```python
from build123d import *

# Parameters (mm, degrees)
EXTRUDE_1_DEPTH             = 8
EXTRUDE_9_DEPTH             = 29
SKETCH_25_W                 = 47
SKETCH_25_H                 = 36.5
EXTRUDE_10_DEPTH            = 4
HOLE_WIZARD_M51_D           = 3.2
HOLE_WIZARD_M51_CBORE_D     = 6
HOLE_WIZARD_M51_CBORE_DEPTH = 35
SKETCH_22_R                 = 2.6
CUT_EXTRUDE_9_DEPTH         = 92.536877814
CUT_EXTRUDE_10_DEPTH        = 4.2
HOLE_WIZARD_M52_D           = 5.2
HOLE_WIZARD_M52_CBORE_D     = 10
HOLE_WIZARD_M52_CBORE_DEPTH = 33
CUT_EXTRUDE_11_DEPTH        = 24
FILLET_1_R                  = 2.5
EXTRUDE_11_DEPTH            = 7
SKETCH_32_W                 = 15
SKETCH_32_H                 = 5.4
CUT_EXTRUDE_12_DEPTH        = 13.5
SKETCH_33_W                 = 15
SKETCH_33_H                 = 5.4
CUT_EXTRUDE_13_DEPTH        = 33.5


with BuildPart() as part:
    # Эскиз1 → Бобышка-Вытянуть1 (new body)
    with BuildSketch(Plane.XY):
        Polygon((-47, 51), (-47, 0), (0, 0), (0, 51), (-22, 51), (-22, 67), (-42, 67), (-42, 51), align=None)
    extrude(amount=EXTRUDE_1_DEPTH)

    # Эскиз24 → Бобышка-Вытянуть9 (add)
    with BuildSketch(Plane.XY.offset(8)):
        with BuildLine():
            Line((0, 51), (-3.5, 51))
            Line((-3.5, 51), (-3.5, 33.5))
            ThreePointArc((-3.5, 33.5), (-13.5, 23.5), (-23.5, 33.5))
            Line((-23.5, 33.5), (-23.5, 51))
            Line((-23.5, 51), (-47, 51))
            Line((-47, 51), (-47, 14.5))
            Line((-47, 14.5), (0, 14.5))
            Line((0, 14.5), (0, 51))
        make_face()
    extrude(amount=EXTRUDE_9_DEPTH)

    # Эскиз25 → Бобышка-Вытянуть10 (add)
    with BuildSketch(Plane.XY.offset(37)):
        with Locations((-23.5, 32.75)):
            Rectangle(SKETCH_25_W, SKETCH_25_H)
    extrude(amount=EXTRUDE_10_DEPTH)

    # Цековка для  болта с шестигранной головкой M51 (through all)
    with Locations(Plane(origin=(-33.5, 3.5, 41), x_dir=(1, 0, 0), z_dir=(0, 0, 1))):
        with Locations((0, 0), (0, 20), (20, 0), (20, 20)):
            CounterBoreHole(HOLE_WIZARD_M51_D / 2, HOLE_WIZARD_M51_CBORE_D / 2, HOLE_WIZARD_M51_CBORE_DEPTH)

    # Эскиз22 → Вырез-Вытянуть9 (cut, through all)
    with BuildSketch(Plane.XY):
        with Locations(Location((-13.5, 33.5, 0), (0, 0, 180))):
            Circle(SKETCH_22_R)
    extrude(amount=CUT_EXTRUDE_9_DEPTH, mode=Mode.SUBTRACT)

    # Эскиз23 → Вырез-Вытянуть10 (cut)
    with BuildSketch(Plane(origin=(0, 0, 0), x_dir=(-1, 0, 0), z_dir=(0, 0, -1))):
        Polygon((13.5, 38.234272207), (9.4, 35.867136104), (9.4, 31.132863896), (13.5, 28.765727793), (17.6, 31.132863896), (17.6, 35.867136104), align=None)
    extrude(amount=-CUT_EXTRUDE_10_DEPTH, mode=Mode.SUBTRACT)

    # Цековка для  болта с шестигранной головкой M52 (through all)
    with Locations(Plane(origin=(-32, 61.5, 41), x_dir=(1, 0, 0), z_dir=(0, 0, 1))):
        with Locations((0, 0), (0, -24.5)):
            CounterBoreHole(HOLE_WIZARD_M52_D / 2, HOLE_WIZARD_M52_CBORE_D / 2, HOLE_WIZARD_M52_CBORE_DEPTH)

    # Эскиз30 → Вырез-Вытянуть11 (cut)
    with BuildSketch(Plane(origin=(0, 51, 0), x_dir=(1, 0, 0), z_dir=(0, 1, 0))):
        Polygon((-42, 0), (-42, -1.2), (-43.2, -1.2), (-44.4, 0), align=None)
        Polygon((-22, 0), (-22, -1.2), (-20.8, -1.2), (-19.6, 0), align=None)
    extrude(amount=-CUT_EXTRUDE_11_DEPTH, mode=Mode.SUBTRACT)

    # Скругление1
    # the kernel refuses this fillet: 2.5 mm, written as the material it adds along each edge
    with BuildSketch(Plane(origin=(-22, 51, -5.05), x_dir=(0, 1, 0), z_dir=(0, 0, 1))) as fillet_1_piece_1_section:
        with BuildLine():
            CenterArc((FILLET_1_R, -FILLET_1_R), FILLET_1_R, 90, 90)
            Line((0, -FILLET_1_R), (0, 0))
            Line((0, 0), (FILLET_1_R, 0))
        make_face()
    fillet_1_piece_1 = extrude(amount=13.05, mode=Mode.PRIVATE)
    fillet_1_piece_1 = split(fillet_1_piece_1, bisect_by=Plane(origin=(-20.123471849, 51.026696565, 0), z_dir=(0, 0, 1)), keep=Keep.TOP, mode=Mode.PRIVATE)
    fillet_1_piece_1 = split(fillet_1_piece_1, bisect_by=Plane(origin=(-20.123471849, 51.026696565, 1.2), z_dir=(0, 0, -1)), keep=Keep.TOP, mode=Mode.PRIVATE)
    fillet_1_piece_1 = split(fillet_1_piece_1, bisect_by=Plane(origin=(-20.293433634, 51.026696565, 0.693433634), z_dir=(0.7071067811865498, 0, 0.7071067811865455)), keep=Keep.TOP, mode=Mode.PRIVATE)
    add(fillet_1_piece_1)
    with BuildSketch(Plane(origin=(-22, 51, 1.2), x_dir=(0, 1, 0), z_dir=(0, 0, 1))) as fillet_1_piece_2_section:
        with BuildLine():
            CenterArc((FILLET_1_R, -FILLET_1_R), FILLET_1_R, 90, 90)
            Line((0, -FILLET_1_R), (0, 0))
            Line((0, 0), (FILLET_1_R, 0))
        make_face()
    fillet_1_piece_2 = extrude(amount=6.8, mode=Mode.PRIVATE)
    fillet_1_piece_2 = split(fillet_1_piece_2, bisect_by=Plane(origin=(-21.509165304, 51.769559816, 1.909165304), z_dir=(-0.7071067811865498, 0, -0.7071067811865455)), keep=Keep.TOP, mode=Mode.PRIVATE)
    add(fillet_1_piece_2)
    with BuildSketch(Plane(origin=(-22, 51, 1.2), x_dir=(0, 1, 0), z_dir=(0, 0, 1))) as fillet_1_piece_3_section:
        with BuildLine():
            CenterArc((FILLET_1_R, -FILLET_1_R), FILLET_1_R, 90, 90)
            Line((0, -FILLET_1_R), (0, 0))
            Line((0, 0), (FILLET_1_R, 0))
        make_face()
    fillet_1_piece_3 = extrude(amount=6.8, mode=Mode.PRIVATE)
    fillet_1_piece_3 = split(fillet_1_piece_3, bisect_by=Plane(origin=(-22.965000899, 51.542951648, 3.365000899), z_dir=(0.7071067811865498, 0, 0.7071067811865455)), keep=Keep.TOP, mode=Mode.PRIVATE)
    add(fillet_1_piece_3)
    with BuildSketch(Plane(origin=(-42, 51, -5.05), x_dir=(0, 1, 0), z_dir=(0, 0, 1))) as fillet_1_piece_4_section:
        with BuildLine():
            CenterArc((FILLET_1_R, FILLET_1_R), FILLET_1_R, 180, 90)
            Line((0, FILLET_1_R), (0, 0))
            Line((0, 0), (FILLET_1_R, 0))
        make_face()
    fillet_1_piece_4 = extrude(amount=13.05, mode=Mode.PRIVATE)
    fillet_1_piece_4 = split(fillet_1_piece_4, bisect_by=Plane(origin=(-43.876528151, 51.026696565, 0), z_dir=(0, 0, 1)), keep=Keep.TOP, mode=Mode.PRIVATE)
    fillet_1_piece_4 = split(fillet_1_piece_4, bisect_by=Plane(origin=(-43.706566366, 51.026696565, 0.693433634), z_dir=(-0.7071067811865488, 0, 0.7071067811865464)), keep=Keep.TOP, mode=Mode.PRIVATE)
    fillet_1_piece_4 = split(fillet_1_piece_4, bisect_by=Plane(origin=(-43.876528151, 51.026696565, 1.2), z_dir=(0, 0, -1)), keep=Keep.TOP, mode=Mode.PRIVATE)
    add(fillet_1_piece_4)
    with BuildSketch(Plane(origin=(-42, 51, 1.2), x_dir=(0, 1, 0), z_dir=(0, 0, 1))) as fillet_1_piece_5_section:
        with BuildLine():
            CenterArc((FILLET_1_R, FILLET_1_R), FILLET_1_R, 180, 90)
            Line((0, FILLET_1_R), (0, 0))
            Line((0, 0), (FILLET_1_R, 0))
        make_face()
    fillet_1_piece_5 = extrude(amount=6.8, mode=Mode.PRIVATE)
    fillet_1_piece_5 = split(fillet_1_piece_5, bisect_by=Plane(origin=(-42.490834696, 51.769559816, 1.909165304), z_dir=(0.7071067811865488, 0, -0.7071067811865464)), keep=Keep.TOP, mode=Mode.PRIVATE)
    add(fillet_1_piece_5)
    with BuildSketch(Plane(origin=(-42, 51, 1.2), x_dir=(0, 1, 0), z_dir=(0, 0, 1))) as fillet_1_piece_6_section:
        with BuildLine():
            CenterArc((FILLET_1_R, FILLET_1_R), FILLET_1_R, 180, 90)
            Line((0, FILLET_1_R), (0, 0))
            Line((0, 0), (FILLET_1_R, 0))
        make_face()
    fillet_1_piece_6 = extrude(amount=6.8, mode=Mode.PRIVATE)
    fillet_1_piece_6 = split(fillet_1_piece_6, bisect_by=Plane(origin=(-41.034999101, 51.542951648, 3.365000899), z_dir=(-0.7071067811865488, 0, 0.7071067811865464)), keep=Keep.TOP, mode=Mode.PRIVATE)
    add(fillet_1_piece_6)
    # the kernel refuses this fillet: 2.5 mm, written as the material it takes off along each edge
    with BuildSketch(Plane(origin=(-47, 0, -6.25), x_dir=(0, 1, 0), z_dir=(0, 0, 1))) as fillet_1_2_piece_1:
        with BuildLine():
            CenterArc((FILLET_1_R, -FILLET_1_R), FILLET_1_R, 90, 90)
            Line((0, -FILLET_1_R), (0, 0))
            Line((0, 0), (FILLET_1_R, 0))
        make_face()
    extrude(amount=20.5, mode=Mode.SUBTRACT)
    with BuildSketch(Plane(origin=(-22, 67, -6.25), x_dir=(-1, 0, 0), z_dir=(0, 0, 1)), Plane(origin=(0, 0, -6.25), x_dir=(0, 1, 0), z_dir=(0, 0, 1)), Plane(origin=(-42, 67, -6.25), x_dir=(0, -1, 0), z_dir=(0, 0, 1))) as fillet_1_2_piece_2:
        with BuildLine():
            CenterArc((FILLET_1_R, FILLET_1_R), FILLET_1_R, 180, 90)
            Line((0, FILLET_1_R), (0, 0))
            Line((0, 0), (FILLET_1_R, 0))
        make_face()
    extrude(amount=20.5, mode=Mode.SUBTRACT)
    with BuildSketch(Plane(origin=(0, 51, 47.25), x_dir=(0, -1, 0), z_dir=(0, 0, -1))) as fillet_1_2_piece_3:
        with BuildLine():
            CenterArc((FILLET_1_R, FILLET_1_R), FILLET_1_R, 180, 90)
            Line((0, FILLET_1_R), (0, 0))
            Line((0, 0), (FILLET_1_R, 0))
        make_face()
    extrude(amount=53.5, mode=Mode.SUBTRACT)
    with BuildSketch(Plane(origin=(-47, 51, 47.25), x_dir=(0, -1, 0), z_dir=(0, 0, -1))) as fillet_1_2_piece_4:
        with BuildLine():
            CenterArc((FILLET_1_R, -FILLET_1_R), FILLET_1_R, 90, 90)
            Line((0, -FILLET_1_R), (0, 0))
            Line((0, 0), (FILLET_1_R, 0))
        make_face()
    extrude(amount=53.5, mode=Mode.SUBTRACT)
    with BuildSketch(Plane(origin=(-47, 14.5, 8), x_dir=(0, 1, 0), z_dir=(0, 0, 1))) as fillet_1_2_piece_5:
        with BuildLine():
            CenterArc((FILLET_1_R, -FILLET_1_R), FILLET_1_R, 90, 90)
            Line((0, -FILLET_1_R), (0, 0))
            Line((0, 0), (FILLET_1_R, 0))
        make_face()
    extrude(amount=39.25, mode=Mode.SUBTRACT)
    with BuildSketch(Plane(origin=(0, 14.5, 8), x_dir=(0, 1, 0), z_dir=(0, 0, 1))) as fillet_1_2_piece_6:
        with BuildLine():
            CenterArc((FILLET_1_R, FILLET_1_R), FILLET_1_R, 180, 90)
            Line((0, FILLET_1_R), (0, 0))
            Line((0, 0), (FILLET_1_R, 0))
        make_face()
    extrude(amount=39.25, mode=Mode.SUBTRACT)

    # Эскиз31 → Бобышка-Вытянуть11 (add)
    with BuildSketch(Plane(origin=(0, 0, 0), x_dir=(-1, 0, 0), z_dir=(0, 0, -1))):
        with BuildLine():
            Line((0, 0), (-9, 0))
            Line((-9, 0), (-9, -4))
            Line((-9, -4), (2.5, -4))
            Line((2.5, -4), (6.5, 0))
            Line((6.5, 0), (2.5, 0))
            ThreePointArc((2.5, 0), (0.732233047, 0.732233047), (0, 2.5))
            Line((0, 2.5), (0, 0))
        make_face()
    extrude(amount=-EXTRUDE_11_DEPTH)

    # Эскиз32 → Вырез-Вытянуть12 (cut)
    with BuildSketch(Plane(origin=(0, 0, 0), x_dir=(0, 0, -1), z_dir=(1, 0, 0))):
        with Locations((-15.5, 26.8)):
            Rectangle(SKETCH_32_W, SKETCH_32_H)
    extrude(amount=-CUT_EXTRUDE_12_DEPTH, mode=Mode.SUBTRACT)

    # Эскиз33 → Вырез-Вытянуть13 (cut)
    with BuildSketch(Plane.ZY.offset(47)):
        with Locations((29.5, 26.8)):
            Rectangle(SKETCH_33_W, SKETCH_33_H)
    extrude(amount=-CUT_EXTRUDE_13_DEPTH, mode=Mode.SUBTRACT)


solid = part.part
```
Source: CAD feature listing. Evaluate the final solid. Frame: model axes, mm. A direction names the side the tool comes from. Coordinates: 2 decimals unless noted, no trailing zeros. Loops run counter-clockwise (first coordinate to the right, second up) from the corner with the lowest first, then second, coordinate; pieces in that order, holes last. Notation, with made-up numbers: (-11.75, -1) - (34.25, -1) arc R14 cw to (34.25, 26) - close; hole circle Ø1 at (68.25, 18.5). An arc over 180 degrees is marked (long way). Answer as CSV lines item,"result".
1. Section C-C (z = 16.5). Return loops of the section in (x, y).
Established:
outline,"(-47, 17) arc R2.5 ccw to (-44.5, 14.5) - (-2.5, 14.5) arc R2.5 ccw to (0, 17) - (0, 24.1) - (-10.09, 24.1) arc R10 cw to (-10.53, 23.95) arc R3 cw (long way) to (-16.47, 23.95) arc R10 cw to (-23.5, 33.5) - (-23.5, 51) - (-44.5, 51) arc R2.5 ccw to (-47, 48.5) - close; (-4.33, 29.5) - (0, 29.5) - (0, 48.5) arc R2.5 ccw to (-2.5, 51) - (-3.5, 51) - (-3.5, 33.5) arc R10 cw to start; hole circle Ø10 at (-32, 37); hole circle Ø6 at (-33.5, 23.5)"
2. Section B-B (z = 36). Return loops of the section in (x, y).
Established:
outline,"(-47, 17) arc R2.5 ccw to (-44.5, 14.5) - (-2.5, 14.5) arc R2.5 ccw to (0, 17) - (0, 48.5) arc R2.5 ccw to (-2.5, 51) - (-3.5, 51) - (-3.5, 33.5) arc R10 cw to (-10.53, 23.95) arc R3 cw (long way) to (-16.47, 23.95) arc R10 cw to (-16.91, 24.1) - (-30.56, 24.1) arc R3 cw (long way) to (-36.44, 24.1) - (-47, 24.1) - close; (-47, 29.5) - (-22.67, 29.5) arc R10 cw to (-23.5, 33.5) - (-23.5, 51) - (-44.5, 51) arc R2.5 ccw to (-47, 48.5) - close; hole circle Ø10 at (-32, 37)"
3. Section D-D (y = 44). Return loops of the section in (x, z), then the cut area to 3 significant figures.
Established:
outline,"(-47, 0) - (-44.4, 0) - (-43.2, 1.2) - (-42, 1.2) - (-42, 0) - (-22, 0) - (-22, 1.2) - (-20.8, 1.2) - (-19.6, 0) - (0, 0) - (0, 41) - (-47, 41) - close; hole (-23.5, 8) - (-3.5, 8) - (-3.5, 37) - (-23.5, 37) - close"
area,"1,340 mm2"
4. Contact query for flat-ended pins moving along their axis: pin 1 (10 mm diameter, centred on y = 49, z = 17.5, fed in from +X); pin 2 (7.5 mm diameter, centred on x = -34, z = 31, fed in from -Y); pin 3 (9.5 mm diameter, centred on x = -13.5, y = 3.5, fed in from +Z); pin 4 (4.5 mm diameter, centred on x = -13.5, y = 33.5, fed in from +Z). Output: stop coordinate, or through.
Established:
pin 1,"stops at x = 0"
pin 2,"stops at y = 14.5"
pin 3,"stops at z = 8"
pin 4,"passes through"
5. Reachability of faces 1 (the flat face through (-9.4, 34, 2)), 2 (the flat face through (-21, 34, 37)), 3 (the flat face through (-32, 2, 6)), 4 (the flat face through (-2, 29.5, 16)), 5 (the flat face through (-24, 24.1, 29)) from +Z, -Z, +X, -X, +Y, -Y: full face, straight path, thin tool, end or side. Return the list, or none.
Established:
face 1,"-Z"
face 2,"none"
face 3,"+Z"
face 4,"+X"
face 5,"-X"
6. Section A-A (y = 3.5). Return loops of the section in (x, z).
Established:
outline,"(-47, 0) - (-35.1, 0) - (-35.1, 6) - (-36.5, 6) - (-36.5, 8) - (-47, 8) - close; (-31.9, 0) - (-15.1, 0) - (-15.1, 6) - (-16.5, 6) - (-16.5, 8) - (-30.5, 8) - (-30.5, 6) - (-31.9, 6) - close; (-11.9, 0) - (0, 0) - (0, 8) - (-10.5, 8) - (-10.5, 6) - (-11.9, 6) - close"
7. Mould query, pull axis X, two halves, no side actions, for faces 6 (the flat face through (-4.5, -2, 3.5)), 7 (the flat face through (-24, 9, 8)), 8 (the cylindrical face through (-36, 40, 25)). Classes: released by +X, released by -X, zero draft, split by the parting line, or undercut.
Established:
face 6,"released by -X"
face 7,"zero draft"
face 8,"undercut"
8. Ray query, line 1 (Z direction, x = -19, y = 45); line 2 (X direction, y = 40.5, z = 13); line 3 (X direction, y = 34.5, z = 33). Return the intervals inside material, ascending.
Established:
line 1,"z = 0 to 8, 37 to 41"
line 2,"x = -47 to -35.57, -28.43 to -23.5, -3.5 to 0"
line 3,"x = -47 to -36.33, -27.67 to -23.5, -3.5 to 0"
